from build123d import *

# Parameters (mm, degrees)
EXTRUDE_1_DEPTH = 2


with BuildPart() as part:
    # Эскиз1 → Бобышка-Вытянуть1 (new body)
    with BuildSketch(Plane(origin=(0, 0, 0), x_dir=(1, 0, 0), z_dir=(0, 1, 0))):
        with BuildLine():
            Line((-0.999103612, 23.957668294), (-1.653583768, 19.471915792))
            ThreePointArc((-1.653583768, 19.471915792), (-2.196840792, 19.142290441), (-2.813399675, 19.29603117))
            Line((-2.813399675, 19.29603117), (-4.78072656, 23.572642625))
            ThreePointArc((-4.78072656, 23.572642625), (-6.018700674, 24.264012159), (-6.703516779, 23.02240085))
            Line((-6.703516779, 23.02240085), (-6.265468091, 18.51036881))
            ThreePointArc((-6.265468091, 18.51036881), (-6.714054544, 18.060311857), (-7.349489911, 18.062032961))
            Line((-7.349489911, 18.062032961), (-10.283109963, 21.743561719))
            ThreePointArc((-10.283109963, 21.743561719), (-11.650566359, 22.118574714), (-12.018345917, 20.749155152))
            Line((-12.018345917, 20.749155152), (-10.513226184, 16.473066476))
            ThreePointArc((-10.513226184, 16.473066476), (-10.841071851, 15.928733595), (-11.458454507, 15.77833505))
            Line((-11.458454507, 15.77833505), (-15.187876393, 18.650824041))
            ThreePointArc((-15.187876393, 18.650824041), (-16.605343475, 18.687686104), (-16.634712476, 17.270043976))
            Line((-16.634712476, 17.270043976), (-14.149993784, 13.478409394))
            ThreePointArc((-14.149993784, 13.478409394), (-14.338045467, 12.871435234), (-14.901495378, 12.577657657))
            Line((-14.901495378, 12.577657657), (-19.209978653, 14.474168263))
            ThreePointArc((-19.209978653, 14.474168263), (-20.595078387, 14.170737105), (-20.28433001, 12.787260619))
            Line((-20.28433001, 12.787260619), (-16.964415179, 9.700436151))
            ThreePointArc((-16.964415179, 9.700436151), (-17.001743998, 9.066095843), (-17.478515502, 8.646012519))
            Line((-17.478515502, 8.646012519), (-22.115666779, 9.456326437))
            ThreePointArc((-22.115666779, 9.456326437), (-23.387902203, 8.830236374), (-22.755096015, 7.561328154))
            Line((-22.755096015, 7.561328154), (-18.792926427, 5.358708819))
            ThreePointArc((-18.792926427, 5.358708819), (-18.677362966, 4.733867916), (-19.039747837, 4.211892561))
            Line((-19.039747837, 4.211892561), (-23.736072739, 3.88891729))
            ThreePointArc((-23.736072739, 3.88891729), (-24.821506154, 2.976554401), (-23.90341855, 1.895958781))
            Line((-23.90341855, 1.895958781), (-19.529261101, 0.705552808))
            ThreePointArc((-19.529261101, 0.705552808), (-19.267521488, 0.126524793), (-19.494459234, -0.467007284))
            Line((-19.494459234, -0.467007284), (-23.977024428, -1.904501593))
            ThreePointArc((-23.977024428, -1.904501593), (-24.81257439, -3.050114094), (-23.662561285, -3.879596824))
            Line((-23.662561285, -3.879596824), (-19.130626105, -3.988607368))
            ThreePointArc((-19.130626105, -3.988607368), (-18.737921695, -4.488171492), (-18.81622352, -5.118766363))
            Line((-18.81622352, -5.118766363), (-22.824518611, -7.587237767))
            ThreePointArc((-22.824518611, -7.587237767), (-23.361625993, -8.899521045), (-22.046521968, -9.429684364))
            Line((-22.046521968, -9.429684364), (-17.620188657, -8.450964181))
            ThreePointArc((-17.620188657, -8.450964181), (-17.119342004, -8.842031563), (-17.044457289, -9.473041346))
            Line((-17.044457289, -9.473041346), (-20.345534735, -12.82903126))
            ThreePointArc((-20.345534735, -12.82903126), (-20.552984809, -14.231720181), (-19.14921893, -14.431752924))
            Line((-19.14921893, -14.431752924), (-15.085729891, -12.422181675))
            ThreePointArc((-15.085729891, -12.422181675), (-14.505848381, -12.682024899), (-14.282129155, -13.2767776))
            Line((-14.282129155, -13.2767776), (-16.684142334, -17.325248088))
            ThreePointArc((-16.684142334, -17.325248088), (-16.549878855, -18.73682347), (-15.139032892, -18.595100462))
            Line((-15.139032892, -18.595100462), (-11.674543338, -15.671467122))
            ThreePointArc((-11.674543338, -15.671467122), (-11.049327577, -15.784985046), (-10.689775588, -16.308915799))
            Line((-10.689775588, -16.308915799), (-12.053128225, -20.814584472))
            ThreePointArc((-12.053128225, -20.814584472), (-11.584954098, -22.153010685), (-10.249021291, -21.677768351))
            Line((-10.249021291, -21.677768351), (-7.584874762, -18.009983863))
            ThreePointArc((-7.584874762, -18.009983863), (-6.950660017, -17.970579237), (-6.476171119, -18.393239092))
            Line((-6.476171119, -18.393239092), (-6.721630115, -23.094252864))
            ThreePointArc((-6.721630115, -23.094252864), (-5.946753919, -24.281745441), (-4.763373826, -23.500603139))
            Line((-4.763373826, -23.500603139), (-3.054400834, -19.301825806))
            ThreePointArc((-3.054400834, -19.301825806), (-2.448045361, -19.111788684), (-1.886195124, -19.408614185))
            Line((-1.886195124, -19.408614185), (-0.999495294, -24.031767224))
            ThreePointArc((-0.999495294, -24.031767224), (0.037049983, -24.999313414), (0.999103612, -23.957668294))
            Line((0.999103612, -23.957668294), (1.653583768, -19.471915792))
            ThreePointArc((1.653583768, -19.471915792), (2.196840792, -19.142290441), (2.813399675, -19.29603117))
            Line((2.813399675, -19.29603117), (4.78072656, -23.572642625))
            ThreePointArc((4.78072656, -23.572642625), (6.018700674, -24.264012159), (6.703516779, -23.02240085))
            Line((6.703516779, -23.02240085), (6.265468091, -18.51036881))
            ThreePointArc((6.265468091, -18.51036881), (6.714054544, -18.060311857), (7.349489911, -18.062032961))
            Line((7.349489911, -18.062032961), (10.283109963, -21.743561719))
            ThreePointArc((10.283109963, -21.743561719), (11.650566359, -22.118574714), (12.018345917, -20.749155152))
            Line((12.018345917, -20.749155152), (10.513226184, -16.473066476))
            ThreePointArc((10.513226184, -16.473066476), (10.841071851, -15.928733595), (11.458454507, -15.77833505))
            Line((11.458454507, -15.77833505), (15.187876393, -18.650824041))
            ThreePointArc((15.187876393, -18.650824041), (16.605343475, -18.687686104), (16.634712476, -17.270043976))
            Line((16.634712476, -17.270043976), (14.149993784, -13.478409394))
            ThreePointArc((14.149993784, -13.478409394), (14.338045467, -12.871435234), (14.901495378, -12.577657657))
            Line((14.901495378, -12.577657657), (19.209978653, -14.474168263))
            ThreePointArc((19.209978653, -14.474168263), (20.595078387, -14.170737105), (20.28433001, -12.787260619))
            Line((20.28433001, -12.787260619), (16.964415179, -9.700436151))
            ThreePointArc((16.964415179, -9.700436151), (17.001743998, -9.066095843), (17.478515502, -8.646012519))
            Line((17.478515502, -8.646012519), (22.115666779, -9.456326437))
            ThreePointArc((22.115666779, -9.456326437), (23.387902203, -8.830236374), (22.755096015, -7.561328154))
            Line((22.755096015, -7.561328154), (18.792926427, -5.358708819))
            ThreePointArc((18.792926427, -5.358708819), (18.677362966, -4.733867916), (19.039747837, -4.211892561))
            Line((19.039747837, -4.211892561), (23.736072739, -3.88891729))
            ThreePointArc((23.736072739, -3.88891729), (24.821506154, -2.976554401), (23.90341855, -1.895958781))
            Line((23.90341855, -1.895958781), (19.529261101, -0.705552808))
            ThreePointArc((19.529261101, -0.705552808), (19.267521488, -0.126524793), (19.494459234, 0.467007284))
            Line((19.494459234, 0.467007284), (23.977024428, 1.904501593))
            ThreePointArc((23.977024428, 1.904501593), (24.81257439, 3.050114094), (23.662561285, 3.879596824))
            Line((23.662561285, 3.879596824), (19.130626105, 3.988607368))
            ThreePointArc((19.130626105, 3.988607368), (18.737921695, 4.488171492), (18.81622352, 5.118766363))
            Line((18.81622352, 5.118766363), (22.824518611, 7.587237767))
            ThreePointArc((22.824518611, 7.587237767), (23.361625993, 8.899521045), (22.046521968, 9.429684364))
            Line((22.046521968, 9.429684364), (17.620188657, 8.450964181))
            ThreePointArc((17.620188657, 8.450964181), (17.119342004, 8.842031563), (17.044457289, 9.473041346))
            Line((17.044457289, 9.473041346), (20.345534735, 12.82903126))
            ThreePointArc((20.345534735, 12.82903126), (20.552984809, 14.231720181), (19.14921893, 14.431752924))
            Line((19.14921893, 14.431752924), (15.085729891, 12.422181675))
            ThreePointArc((15.085729891, 12.422181675), (14.505848381, 12.682024899), (14.282129155, 13.2767776))
            Line((14.282129155, 13.2767776), (16.684142334, 17.325248088))
            ThreePointArc((16.684142334, 17.325248088), (16.549878855, 18.73682347), (15.139032892, 18.595100462))
            Line((15.139032892, 18.595100462), (11.674543338, 15.671467122))
            ThreePointArc((11.674543338, 15.671467122), (11.049327577, 15.784985046), (10.689775588, 16.308915799))
            Line((10.689775588, 16.308915799), (12.053128225, 20.814584472))
            ThreePointArc((12.053128225, 20.814584472), (11.584954098, 22.153010685), (10.249021291, 21.677768351))
            Line((10.249021291, 21.677768351), (7.584874762, 18.009983863))
            ThreePointArc((7.584874762, 18.009983863), (6.950660017, 17.970579237), (6.476171119, 18.393239092))
            Line((6.476171119, 18.393239092), (6.721630115, 23.094252864))
            ThreePointArc((6.721630115, 23.094252864), (5.946753919, 24.281745441), (4.763373826, 23.500603139))
            Line((4.763373826, 23.500603139), (3.054400834, 19.301825806))
            ThreePointArc((3.054400834, 19.301825806), (2.448045361, 19.111788684), (1.886195124, 19.408614185))
            Line((1.886195124, 19.408614185), (0.999495294, 24.031767224))
            ThreePointArc((0.999495294, 24.031767224), (-0.037049983, 24.999313414), (-0.999103612, 23.957668294))
        make_face()
        Polygon((4.960496045, -6.38175621), (8.007011021, 1.105037486), (3.046514976, 7.486793695), (-4.960496045, 6.38175621), (-8.007011021, -1.105037486), (-3.046514976, -7.486793695), align=None, mode=Mode.SUBTRACT)
    extrude(amount=EXTRUDE_1_DEPTH)


solid = part.part
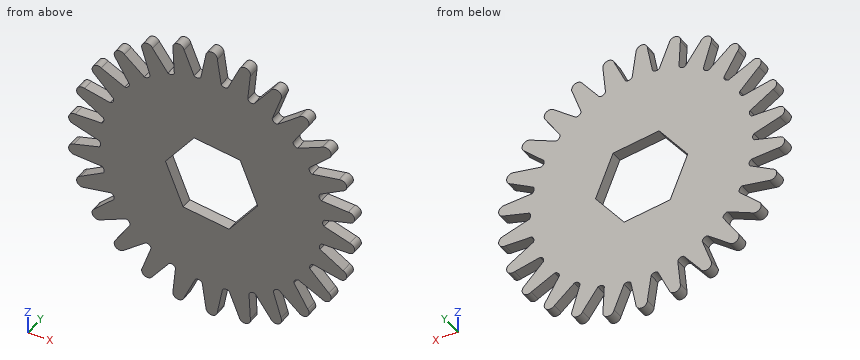
The listing builds one solid part. Answer for the finished solid, in the listing's coordinates (mm). Round coordinates to 2 decimals unless told otherwise and drop trailing zeros. Order: outer loops, then holes, each group sorted by start corner. A loop starts at its lowest first (then second) coordinate and runs counter-clockwise, first axis right, second up. Notation, with made-up numbers: M 15,36 L 53,36 A26 cw 53,50 Z; hole C 39.25,-4 d6. An arc over 180 degrees is marked long. Answer in a Markdown table with one row per item. Add a question column.
1) A flat-ended cylindrical pin translates along its axis: pin 1 Ø1 at (x, y) = (15.5, 0.5) entering from +Z. Find the tip coordinate at first contact, or state that the pin passes through.
2) The part is cut by section A-A on x = 0. Determine the outline of the cut face in (y, z).
3) The part is cut by section B-B on x = 13.5. Determine the outline of the cut face in (y, z).
4) Consider line 1 along X through (y, z) = (0.9, -19); line 2 along X through (y, z) = (1.85, -22); line 3 along Z through (x, y) = (-21, 1.5). Determine where each line is inside the solid, lowest interval first. Write a range as from..to.
5) The part is cut by section C-C on x = -13. Determine the outline of the cut face in (y, z).
Findings below:
| question | item | result |
|---|---|---|
| 1 | pin 1 | stops at z = 18.96 |
| 2 | outline | M 0,-25 L 2,-25 L 2,-7.07 L 0,-7.07 Z; M 0,7.07 L 2,7.07 L 2,25 L 0,25 Z |
| 3 | outline | M 0,-17.21 L 2,-17.21 L 2,17.35 L 0,17.35 Z |
| 4 | line 1 | x = -11.4..-8.1, -6.31..6.51, 8.3..11.5 |
| 4 | line 2 | x = -11.82..-10.49, -6.6..-4.06, -1.28..1.39, 4.15..6.66, 10.49..11.82 |
| 4 | line 3 | z = -9.26..-6.59, -4.08..-1.11, 0.95..3.94, 6.46..9.2 |
| 5 | outline | M 0,-16.97 L 2,-16.97 L 2,16.79 L 0,16.79 Z |
